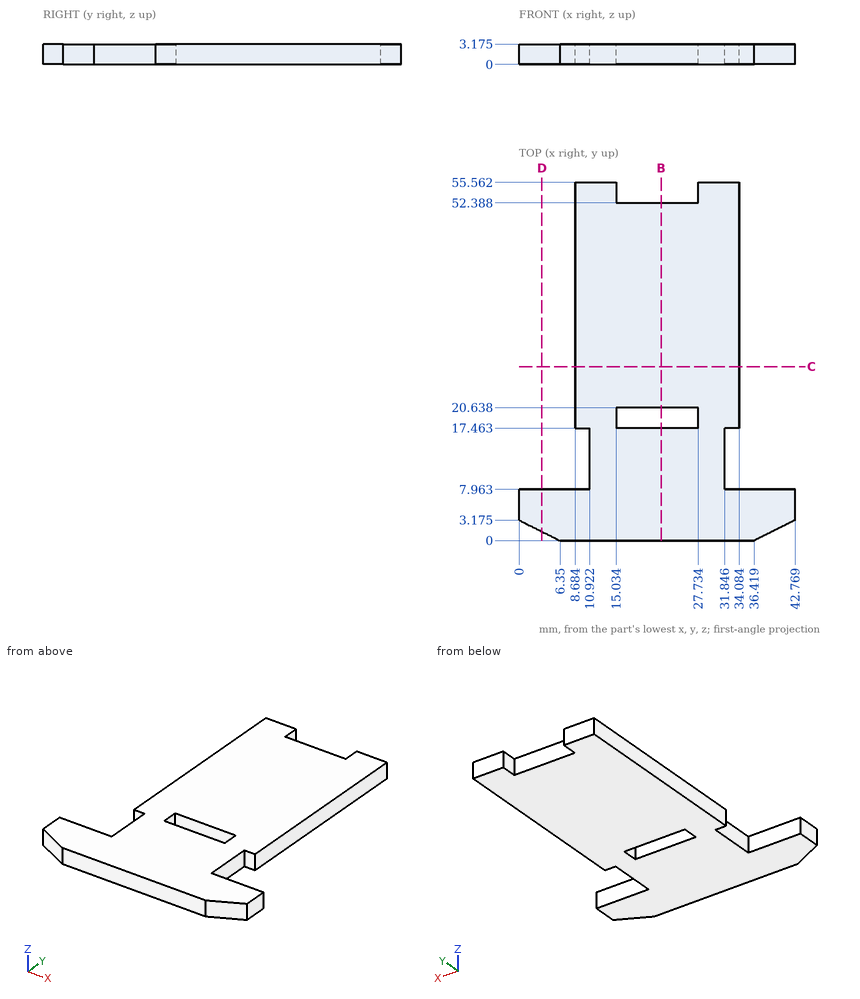
Answer from the drawing. Dimensions are ordinates in mm from the lowest x, y and z of the part. Coordinates: 2 decimals unless noted, no trailing zeros. Write each loop counter-clockwise with the first axis right and the second up, starting at its lowest first coordinate (ties: lowest second). Pieces come first, ordered by that corner, then holes. Notation, with made-up numbers: M -24.5,24.5 L -7.5,24.5 A32 ccw -7.5,54.5 Z; hole C 78,7.25 d11. An arc over 180 degrees is marked long. Put each result on its own line as item: value. Start each with the question number.
1. A cutting plane is placed at B-B on x = 22. Write down the section's boundary in (y, z) (1 decimal).
2. Consider line 1 (Y direction, x = 23.5, z = 2.3); line 2 (X direction, y = 52.5, z = 0.25) (1 decimal); line 3 (X direction, y = 30, z = 1.3) (1 decimal). Determine where each line is inside the solid, lowest interval first. Write a range as from..to.
3. A cutting plane is placed at C-C on y = 27. Write down the section's boundary in (x, z) (1 decimal).
4. Flat-ended cylindrical pins translate along their axes: P1, Ø1.6, axis at y = 32, z = 1, coming from the -X side; P2, Ø1.6, axis at y = 32, z = 1.5, coming from the +X side; P3, Ø6, axis at x = 32.5, y = 38.5, coming from the -Z side; P4, Ø1, axis at x = 21, z = 1, coming from the +Y side. Find the tip coordinate at first contact, or state that the pin passes through.
5. A cutting plane is placed at D-D on x = 3.5. Write down the section's boundary in (y, z) (1 decimal).
Resolved:
1. outline: M 0,0 L 17.5,0 L 17.5,3.2 L 0,3.2 Z; M 20.6,0 L 52.4,0 L 52.4,3.2 L 20.6,3.2 Z
2. line 1: y = 0..17.46, 20.64..52.39
2. line 2: x = 8.7..15, 27.7..34.1
2. line 3: x = 8.7..34.1
3. outline: M 8.7,0 L 34.1,0 L 34.1,3.2 L 8.7,3.2 Z
4. P1: stops at x = 8.68
4. P2: stops at x = 34.08
4. P3: stops at z = 0
4. P4: stops at y = 52.39
5. outline: M 1.4,0 L 8,0 L 8,3.2 L 1.4,3.2 Z
